Verification items for the finished model (mm, model axes). A direction names the side the tool comes from. Give positions to 0.01 mm unless a question says otherwise; leave off trailing zeros. Order: outer loops, then holes, each group sorted by start corner. A loop starts at its lowest first (then second) coordinate and runs counter-clockwise, first axis right, second up. Notation, with made-up numbers: (89, 68) - (148, 68) arc R30 cw to (148, 96) - close; hole circle Ø2 at (-12.75, 88). An arc over 180 degrees is marked (long way). Answer as a JSON object with one key per item and string values.
```python
from build123d import *

# Parameters (mm, degrees)
SKETCH1_W             = 62
SKETCH1_H             = 123
EXTRUDE1_DEPTH        = 5
SKETCH2_W             = 38
SKETCH2_H             = 5
EXTRUDE2_DEPTH        = 25
SKETCH3_W             = 86
SKETCH3_H             = 5
EXTRUDE3_DEPTH        = 26
SKETCH4_W             = 86
SKETCH4_H             = 5
EXTRUDE4_DEPTH        = 26
LPATTERN1_COUNT       = 2
LPATTERN1_PITCH       = 25
LPATTERN1_COUNT_DIR2  = 2
LPATTERN1_PITCH_DIR2  = 50
M3X0_5_TAPPED_HOLE1_D = 2.5
LPATTERN2_COUNT       = 2
LPATTERN2_PITCH       = 22.9


with BuildPart() as part:
    # Sketch1 → Extrude1 (new body)
    with BuildSketch(Plane(origin=(0, 0, 0), x_dir=(1, 0, 0), z_dir=(0, 1, 0))):
        Rectangle(SKETCH1_W, SKETCH1_H)
    extrude(amount=EXTRUDE1_DEPTH)

    # Sketch2 → Extrude2 (cut)
    with BuildSketch(Plane(origin=(0, 0, -61.5), x_dir=(-1, 0, 0), z_dir=(0, 0, -1))):
        with Locations((0, 2.5)):
            Rectangle(SKETCH2_W, SKETCH2_H)
    extrude(amount=-EXTRUDE2_DEPTH, mode=Mode.SUBTRACT)

    # Sketch3 → Extrude3 (cut)
    with BuildSketch(Plane.ZY.offset(31)):
        with Locations((18.5, 2.5)):
            Rectangle(SKETCH3_W, SKETCH3_H)
    extrude(amount=-EXTRUDE3_DEPTH, mode=Mode.SUBTRACT)

    # Sketch4 → Extrude4 (cut)
    with BuildSketch(Plane(origin=(31, 0, 0), x_dir=(0, 0, -1), z_dir=(1, 0, 0))):
        with Locations((-18.5, 2.5)):
            Rectangle(SKETCH4_W, SKETCH4_H)
    extrude(amount=-EXTRUDE4_DEPTH, mode=Mode.SUBTRACT)

    # Sketch6 → M6 Clearance Hole1 (revolve, cut)
    with BuildSketch(Plane(origin=(-25, 5, -55.5), x_dir=(0, 0, 1), z_dir=(1, 0, 0))):
        Polygon((0, 0), (0, 11.982840043), (3.3, 10), (3.3, 0), align=None)
    m6_clearance_hole1 = revolve(axis=Axis((-25, 11.35, -55.5), (0, -1, 0)), mode=Mode.SUBTRACT)

    # LPattern1: M6 Clearance Hole1 2 × 2
    with Locations(*[(j * LPATTERN1_PITCH_DIR2, 0, i * LPATTERN1_PITCH) for i in range(LPATTERN1_COUNT) for j in range(LPATTERN1_COUNT_DIR2) if (i, j) != (0, 0)]):
        add(m6_clearance_hole1, mode=Mode.SUBTRACT)

    # M3x0.5 Tapped Hole1 (through all)
    with Locations(Plane(origin=(0, 5, 58.5), x_dir=(0, 0, 1), z_dir=(0, 1, 0))):
        with Locations((0, 0)):
            m3x0_5_tapped_hole1 = Hole(M3X0_5_TAPPED_HOLE1_D / 2)

    # LPattern2: M3x0.5 Tapped Hole1 ×2
    with Locations(*[(0, 0, -i * LPATTERN2_PITCH) for i in range(1, LPATTERN2_COUNT)]):
        add(m3x0_5_tapped_hole1, mode=Mode.SUBTRACT)


solid = part.part
```
(1) Material ranges on line 1 along X through (y, z) = (2.75, -30.5); line 2 along Z through (x, y) = (25, 3.85); line 3 along X through (y, z) = (1.5, -47.5), recorded low to high. Write a range as [from, to].
Computed values:
{"line 1": "x = [-31, -28.3], [-21.7, 21.7], [28.3, 31]", "line 2": "z = [-61.5, -58.8], [-52.2, -33.8], [-27.2, -24.5]", "line 3": "x = [-31, -19], [19, 31]"}
(2) Section check C-C (z = -40.5). Record the cut outline in (x, y), then the cut area to 3 significant figures.
Computed values:
{"outline": "(-31, 0) - (-19, 0) - (-19, 5) - (-31, 5) - close; (19, 0) - (31, 0) - (31, 5) - (19, 5) - close", "area": "120 mm²"}
(3) Gauge pin test, flat end, axial feed: pin 1 Ø2.5 at (x, y) = (-18.5, 2.5) entering from +Z. Record the tip position at first contact, or that the pin passes through.
Computed values:
{"pin 1": "stops at z = -24.5"}
(4) Section check D-D (y = 1.8). Record the cut outline in (x, z).
Computed values:
{"outline": "(-31, -61.5) - (-19, -61.5) - (-19, -36.5) - (19, -36.5) - (19, -61.5) - (31, -61.5) - (31, -24.5) - (5, -24.5) - (5, 61.5) - (-5, 61.5) - (-5, -24.5) - (-31, -24.5) - close; hole circle Ø6.6 at (-25, -55.5); hole circle Ø6.6 at (-25, -30.5); hole circle Ø2.5 at (0, 35.6); hole circle Ø2.5 at (0, 58.5); hole circle Ø6.6 at (25, -55.5); hole circle Ø6.6 at (25, -30.5)"}
(5) Release check for a two-part mould opening along Z. For faces 1 (the flat face through (-25, 2, -61.5)), 2 (the cylindrical face through (0.38, 2.47, 57.31)), 3 (the flat face through (-19, 2, -49)), 4 (the cylindrical face through (24.9, 2.5, -58.8)) record: pulls with the +Z half, pulls with the -Z half, needs draft (parallel to the pull), parting line crosses it, or undercut.
Computed values:
{"face 1": "pulls with the -Z half", "face 2": "undercut", "face 3": "needs draft", "face 4": "undercut"}
(6) Access from +Z, -Z, +X, -X, +Y, -Y to the whole of each face (thin tool, end or side, straight path). Record for faces 5 (the flat face through (19, 2, -49)), 6 (the cylindrical face through (0.38, 2.47, 34.41)), 7 (the flat face through (18, 2, -24.5)), 8 (the flat face through (0, 0, -14)), 9 (the flat face through (-18, 2, -24.5)).
Computed values:
{"face 5": "-Z, +Y, -Y", "face 6": "+Y, -Y", "face 7": "+Z, +X, +Y, -Y", "face 8": "+Z, -Z, +X, -X, -Y", "face 9": "+Z, -X, +Y, -Y"}
(7) Section check A-A (x = 25). Record the cut outline in (y, z).
Computed values:
{"outline": "(0, -61.5) - (5, -61.5) - (5, -58.8) - (0, -58.8) - close; (0, -52.2) - (5, -52.2) - (5, -33.8) - (0, -33.8) - close; (0, -27.2) - (5, -27.2) - (5, -24.5) - (0, -24.5) - close"}
(8) Section check B-B (z = -55.5). Record the cut outline in (x, y).
Computed values:
{"outline": "(-31, 0) - (-28.3, 0) - (-28.3, 5) - (-31, 5) - close; (-21.7, 0) - (-19, 0) - (-19, 5) - (-21.7, 5) - close; (19, 0) - (21.7, 0) - (21.7, 5) - (19, 5) - close; (28.3, 0) - (31, 0) - (31, 5) - (28.3, 5) - close"}
